```python
from build123d import *

# Parameters (mm, degrees)
SKETCH2_R           = 39.5
BOSS_EXTRUDE1_DEPTH = 1
SKETCH4_R           = 41.25
BOSS_EXTRUDE2_DEPTH = 1
SKETCH5_R           = 42
BOSS_EXTRUDE3_DEPTH = 7
SKETCH6_R           = 35
BOSS_EXTRUDE4_DEPTH = 7
BOSS_EXTRUDE5_DEPTH = 3
CIRPATTERN1_COUNT   = 12
SKETCH8_R           = 15
BOSS_EXTRUDE6_DEPTH = 10
SKETCH9_W           = 20
SKETCH9_H           = 40
BOSS_EXTRUDE7_DEPTH = 42
BOSS_EXTRUDE8_DEPTH = 20
SKETCH11_R          = 15
BOSS_EXTRUDE9_DEPTH = 10


with BuildPart() as part:
    # Sketch1 → Revolve1 (revolve)
    with BuildSketch(Plane.XY):
        with BuildLine():
            Line((-35, 0), (0, 0))
            Line((0, 0), (0, -20))
            Line((0, -20), (-40, -20))
            ThreePointArc((-40, -20), (-39.657515479, -9.46062113), (-35, 0))
        make_face()
    revolve(axis=Axis((0, 0, 0), (0, -1, 0)))

    # Sketch2 → Boss-Extrude1 (add)
    with BuildSketch(Plane.XZ.offset(20)):
        Circle(SKETCH2_R)
    extrude(amount=BOSS_EXTRUDE1_DEPTH)

    # Sketch3 → Revolve2 (revolve)
    with BuildSketch(Plane(origin=(0, 0, 0), x_dir=(0, 0, -1), z_dir=(1, 0, 0)), mode=Mode.PRIVATE) as revolve2_sk:
        with BuildLine():
            Line((0, -21), (-40, -21))
            ThreePointArc((-40, -21), (-42.384109041, -30.861589096), (-42, -41))
            Line((-42, -41), (0, -41))
            Line((0, -41), (0, -21))
        make_face()
    revolve(revolve2_sk.sketch.rotate(Axis((0, -21, 0), (0, -1, 0)), 90), axis=Axis((0, -21, 0), (0, -1, 0)))

    # Sketch4 → Boss-Extrude2 (add)
    with BuildSketch(Plane.XZ.offset(41)):
        with Locations(Location((0, 0, 0), (0, 0, 270))):
            Circle(SKETCH4_R)
    extrude(amount=BOSS_EXTRUDE2_DEPTH)

    # Sketch5 → Boss-Extrude3 (add)
    with BuildSketch(Plane.XZ.offset(42)):
        with Locations(Location((0, 0, 0), (0, 0, 270))):
            Circle(SKETCH5_R)
    extrude(amount=BOSS_EXTRUDE3_DEPTH)

    # Sketch6 → Boss-Extrude4 (add)
    with BuildSketch(Plane.XZ.offset(49)):
        with Locations(Location((0, 0, 0), (0, 0, 270))):
            Circle(SKETCH6_R)
    extrude(amount=BOSS_EXTRUDE4_DEPTH)

    # Sketch7 → Boss-Extrude5 (add)
    with BuildSketch(Plane.XZ.offset(49)):
        Polygon((40.75, 0), (39.625, 1.948557159), (37.375, 1.948557159), (36.25, 0), (37.375, -1.948557159), (39.625, -1.948557159), align=None)
        Polygon((39.047649731, 0.948557159), (37.952350269, 0.948557159), (37.404700538, 0), (37.952350269, -0.948557159), (39.047649731, -0.948557159), (39.595299462, 0), align=None, mode=Mode.SUBTRACT)
    boss_extrude5 = extrude(amount=BOSS_EXTRUDE5_DEPTH)

    # CirPattern1: Boss-Extrude5 ×12 about axis
    cirpattern1_axis = Axis((0, 0, 0), (0, 1, 0))
    for i in range(1, CIRPATTERN1_COUNT):
        add(boss_extrude5.rotate(cirpattern1_axis, i * 360 / CIRPATTERN1_COUNT))

    # Sketch8 → Boss-Extrude6 (add)
    with BuildSketch(Plane.XZ.offset(56)):
        with Locations(Location((0, 0, 0), (0, 0, 270))):
            Circle(SKETCH8_R)
    extrude(amount=BOSS_EXTRUDE6_DEPTH)

    # Sketch9 → Boss-Extrude7 (add)
    with BuildSketch(Plane(origin=(0, 0, 0), x_dir=(1, 0, 0), z_dir=(0, 1, 0))):
        Rectangle(SKETCH9_W, SKETCH9_H)
    extrude(amount=BOSS_EXTRUDE7_DEPTH)

    # Sketch10 → Boss-Extrude8 (add)
    with BuildSketch(Plane.ZY.offset(10)):
        with BuildLine():
            Line((-20, 42), (20, 42))
            ThreePointArc((20, 42), (0, 62), (-20, 42))
        make_face()
    extrude(amount=-BOSS_EXTRUDE8_DEPTH)

    # Sketch11 → Boss-Extrude9 (add)
    with BuildSketch(Plane.ZY.offset(10)):
        with Locations(Location((0, 42, 0), (0, 0, 90))):
            Circle(SKETCH11_R)
    boss_extrude9 = extrude(amount=BOSS_EXTRUDE9_DEPTH)

    # Mirror1: Boss-Extrude9 across plane
    add(boss_extrude9.mirror(Plane(origin=(0, 0, 0), x_dir=(0, 0, 1), z_dir=(1, 0, 0))))


solid = part.part
```
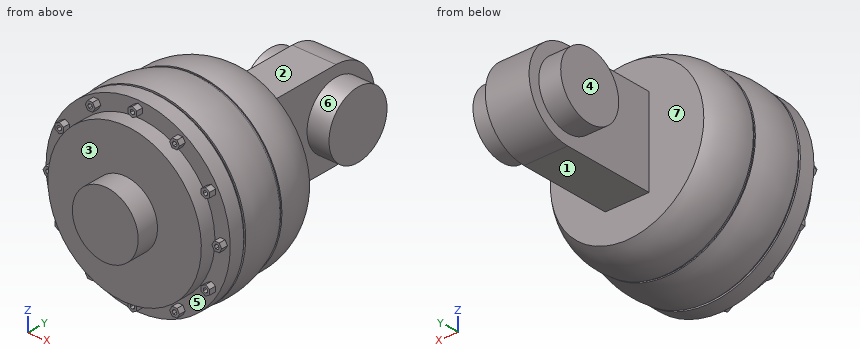
Here's how the part is built. I have some questions about the finished solid (model axes, mm). Face numbers are marked on the shaded views. A direction names the side the tool comes from. Coordinates: 2 decimals unless noted, no trailing zeros. Order: outer loops, then holes, each group sorted by start corner. A loop starts at its lowest first (then second) coordinate and runs counter-clockwise, first axis right, second up.
Item 1: If we section it at A-A, the plane y = 39: List the corners of the cut face in (x, z) for me, then the cut area to 3 significant figures.
Response values:
outline: (-20, -14.7) - (-10, -14.7) - (-10, -20) - (10, -20) - (10, -14.7) - (20, -14.7) - (20, 14.7) - (10, 14.7) - (10, 20) - (-10, 20) - (-10, 14.7) - (-20, 14.7) - close
area: 1,390 mm2
Item 2: Which directions (+Z, -Z, +X, -X, +Y, -Y) give clear straight access to the entire face, cutting with the end or side of a thin tool? Please do the marked faces 1, 2 and 3.
Response values:
face 1: -Z, +X, -X, +Y
face 2: +Z, +X, -X, +Y
face 3: -Y
Item 3: Thinking about a two-plate mould opening in Y: for the marked faces 4, 5, 6 and 7, which applies, pulls with the +Y half, pulls with the -Y half, needs draft (parallel to the pull), parting line crosses it, or undercut?
Response values:
face 4: needs draft
face 5: pulls with the -Y half
face 6: undercut
face 7: undercut
Item 4: If we section it at B-B, the plane y = 14: List the corners of the cut face in (x, z) for me, then the cut area to 3 significant figures.
Response values:
outline: (-10, -20) - (10, -20) - (10, 20) - (-10, 20) - close
area: 800 mm2
Item 5: I need wall thicknesses on probe 1 along Y at (x, z) = (-22.5, 10); probe 2 along X at (y, z) = (24, 15.5); probe 3 along Y at (x, z) = (-13, -5). Which ranges of each line are inside material? Lowest first, please.
Response values:
probe 1: y = -56 to 0
probe 2: x = -10 to 10
probe 3: y = -66 to 0, 27.86 to 56.14
Item 6: I'm going to push flat-ended pins straight in: pin 1 Ø4 at (y, z) = (-9, -28) entering from +X; pin 2 Ø12 at (y, z) = (19, 3) entering from -X; pin 3 Ø0.5 at (y, z) = (-50.5, 38.5) entering from +X. Where does each tip first touch, or does it pass through?
Response values:
pin 1: stops at x = 29.91
pin 2: stops at x = -10
pin 3: stops at x = 1.95
